Source: CAD feature listing. Evaluate the final solid. Frame: model axes, mm. Round coordinates to 2 decimals unless told otherwise and drop trailing zeros. Order: outer loops, then holes, each group sorted by start corner. A loop starts at its lowest first (then second) coordinate and runs counter-clockwise, first axis right, second up. Notation, with made-up numbers: (-29, 60.25) -> (19, 60.25) arc R14 ccw to (19, 75.25) -> close; hole circle Ø11 at (51.25, 50). An arc over 180 degrees is marked (long way). Write item = value, one per line. Start each with the question number.
(1) Cut plane B-B on x = -16. Return the cut outline in (y, z).
(2) Ray query, line 1 (Y direction, x = -49.5, z = 0.55); line 2 (Y direction, x = -12, z = 0.85); line 3 (Y direction, x = -76.5, z = 0.15). Return the intervals inside material, ascending.
(3) Contact query for flat-ended pins moving along their axis: pin 1 Ø1 at (y, z) = (76.5, 1) entering from +X; pin 2 Ø1 at (y, z) = (39, 1) entering from +X; pin 3 Ø1 at (y, z) = (20, 1.5) entering from -X. Output: stop coordinate, or through.
(4) Cut plane A-A on x = -49. Return the cut outline in (y, z).
(5) Cut plane C-C on y = 42. Give the number of separate pieces and of enclosed holes in the cut face, then the cut area to 3 significant figures.
from build123d import *

# Parameters (mm, degrees)
F2_DEPTH = 2
F3_W     = 2
F3_H     = 10
F3_H_2   = 7.419568
F4_DEPTH = 25
F6_DEPTH = 2
F7_W     = 5
F7_H     = 44.93185
F7_H_2   = 80.277377
F7_H_3   = 143.82022
F7_H_4   = 146.914949
F7_H_5   = 150.008155
F7_H_6   = 155.922672
F7_H_7   = 152.60311
F7_H_8   = 158.631397
F7_H_9   = 74.565352
F7_H_10  = 59.935174
F7_H_11  = 17.802537
F7_H_12  = 20.475702
F7_H_13  = 22.61665
F7_H_14  = 22.198746
F7_H_15  = 21.923671
F7_H_16  = 21.644043
F7_H_17  = 21.303791
F7_H_18  = 21.036336
F7_H_19  = 20.777645
F7_H_20  = 20.346487
F7_W_2   = 3
F7_H_21  = 20.140204
F8_DEPTH = 5


with BuildPart() as f2:
    # F1 (on Top) → F2 (new body)
    with BuildSketch(Plane.XY):
        with BuildLine():
            Line((-10.286918, 88.926369), (-80.9691, 88.926369))
            Line((-80.9691, 88.926369), (-80.9691, -91.073631))
            Line((-80.9691, -91.073631), (79.0309, -91.073631))
            Line((79.0309, -91.073631), (79.0309, -62.904311))
            Line((79.0309, -62.904311), (-0.788567, -58.895134))
            ThreePointArc((-0.788567, -58.895134), (-7.533175, -55.799151), (-10.286918, -48.907724))
            Line((-10.286918, -48.907724), (-10.286918, 88.926369))
        make_face()
    extrude(amount=F2_DEPTH)

    # F3 (on Top) → F4 (cut)
    with BuildSketch(Plane.XY):
        Polygon((-10.970959, -7.614357), (-20.367885, -11.034559), (-19.683845, -12.913944), (-10.286918, -9.493742), align=None)
        Polygon((-5.092329, -5.474711), (-10.970959, -7.614357), (-10.286918, -9.493742), (-4.408289, -7.354096), align=None)
        Polygon((-10.970959, 80.805754), (-20.367885, 77.385553), (-19.683845, 75.506168), (-10.286918, 78.926369), align=None)
        Polygon((-3.998845, 83.343396), (-10.970959, 80.805754), (-10.286918, 78.926369), (-3.314805, 81.464011), align=None)
        Polygon((-80.9691, 32.230381), (-71.572174, 28.810179), (-70.888133, 30.689565), (-80.28506, 34.109766), align=None)
        Polygon((-87.941213, 34.768023), (-80.9691, 32.230381), (-80.28506, 34.109766), (-87.257173, 36.647408), align=None)
        Polygon((-80.9691, -61.360746), (-71.572174, -64.780947), (-70.888133, -62.901562), (-80.28506, -59.48136), align=None)
        Polygon((-87.941213, -58.823104), (-80.9691, -61.360746), (-80.28506, -59.48136), (-87.257173, -56.943719), align=None)
        with Locations((75.0309, -67.753627)):
            Rectangle(F3_W, F3_H)
        with Locations((75.0309, -59.043843)):
            Rectangle(F3_W, F3_H_2)
    extrude(amount=F4_DEPTH, mode=Mode.SUBTRACT)

    # F5 (on Top) → F6 (join)
    with BuildSketch(Plane.XY):
        with BuildLine():
            Line((-84.190791, -61.073631), (-86.1691, -61.073631))
            ThreePointArc((-86.1691, -61.073631), (-87.583313, -61.659417), (-88.1691, -63.073631))
            Line((-88.1691, -63.073631), (-88.1691, -79.073631))
            ThreePointArc((-88.1691, -79.073631), (-87.583313, -80.487844), (-86.1691, -81.073631))
            Line((-86.1691, -81.073631), (-83.1691, -81.073631))
            Line((-83.1691, -81.073631), (-80.9691, -81.073631))
            Line((-80.9691, -81.073631), (-80.9691, -71.073631))
            Line((-80.9691, -71.073631), (-83.1691, -71.073631))
            Line((-83.1691, -71.073631), (-83.1691, -62.095322))
            ThreePointArc((-83.1691, -62.095322), (-83.468346, -61.372877), (-84.190791, -61.073631))
        make_face()
        with BuildLine():
            Line((-84.190791, 18.926369), (-86.1691, 18.926369))
            ThreePointArc((-86.1691, 18.926369), (-87.583313, 18.340583), (-88.1691, 16.926369))
            Line((-88.1691, 16.926369), (-88.1691, 0.926369))
            ThreePointArc((-88.1691, 0.926369), (-87.583313, -0.487844), (-86.1691, -1.073631))
            Line((-86.1691, -1.073631), (-83.1691, -1.073631))
            Line((-83.1691, -1.073631), (-80.9691, -1.073631))
            Line((-80.9691, -1.073631), (-80.9691, 8.926369))
            Line((-80.9691, 8.926369), (-83.1691, 8.926369))
            Line((-83.1691, 8.926369), (-83.1691, 17.904678))
            ThreePointArc((-83.1691, 17.904678), (-83.468346, 18.627123), (-84.190791, 18.926369))
        make_face()
        with BuildLine():
            Line((-84.190791, 83.926369), (-86.1691, 83.926369))
            ThreePointArc((-86.1691, 83.926369), (-87.583313, 83.340583), (-88.1691, 81.926369))
            Line((-88.1691, 81.926369), (-88.1691, 65.926369))
            ThreePointArc((-88.1691, 65.926369), (-87.583313, 64.512156), (-86.1691, 63.926369))
            Line((-86.1691, 63.926369), (-80.9691, 63.926369))
            Line((-80.9691, 63.926369), (-80.9691, 73.926369))
            Line((-80.9691, 73.926369), (-83.1691, 73.926369))
            Line((-83.1691, 73.926369), (-83.1691, 82.904678))
            ThreePointArc((-83.1691, 82.904678), (-83.468346, 83.627123), (-84.190791, 83.926369))
        make_face()
        with BuildLine():
            Line((-10.286918, 58.926369), (-9.800001, 58.926369))
            Line((-9.800001, 58.926369), (-8.086918, 58.926369))
            Line((-8.086918, 58.926369), (-7.600001, 58.926369))
            Line((-7.600001, 58.926369), (-5.086918, 58.926369))
            ThreePointArc((-5.086918, 58.926369), (-3.672705, 59.512156), (-3.086918, 60.926369))
            Line((-3.086918, 60.926369), (-3.086918, 76.926369))
            ThreePointArc((-3.086918, 76.926369), (-3.672705, 78.340583), (-5.086918, 78.926369))
            Line((-5.086918, 78.926369), (-7.065227, 78.926369))
            ThreePointArc((-7.065227, 78.926369), (-7.787672, 78.627123), (-8.086918, 77.904678))
            Line((-8.086918, 77.904678), (-8.086918, 68.926369))
            Line((-8.086918, 68.926369), (-10.286918, 68.926369))
            Line((-10.286918, 68.926369), (-10.286918, 58.926369))
        make_face()
        with BuildLine():
            Line((-10.286918, -21.073631), (-10.286918, -31.073631))
            Line((-10.286918, -31.073631), (-8.086918, -31.073631))
            Line((-8.086918, -31.073631), (-5.086918, -31.073631))
            ThreePointArc((-5.086918, -31.073631), (-3.672705, -30.487844), (-3.086918, -29.073631))
            Line((-3.086918, -29.073631), (-3.086918, -13.073631))
            ThreePointArc((-3.086918, -13.073631), (-3.672705, -11.659417), (-5.086918, -11.073631))
            Line((-5.086918, -11.073631), (-7.065227, -11.073631))
            ThreePointArc((-7.065227, -11.073631), (-7.787672, -11.372877), (-8.086918, -12.095322))
            Line((-8.086918, -12.095322), (-8.086918, -21.073631))
            Line((-8.086918, -21.073631), (-10.286918, -21.073631))
        make_face()
    extrude(amount=F6_DEPTH)

    # F7 (on Top) → F8 (cut)
    with BuildSketch(Plane.XY):
        with Locations((-73.4691, 61.460444)):
            Rectangle(F7_W, F7_H)
        with Locations((-72.413613, -17.006834)):
            Rectangle(F7_W, F7_H_2)
        with Locations((-65.4691, 12.016259)):
            Rectangle(F7_W, F7_H_3)
        with Locations((-57.4691, 10.468894)):
            Rectangle(F7_W, F7_H_4)
        with Locations((-49.4691, 8.922292)):
            Rectangle(F7_W, F7_H_5)
        with Locations((-33.4691, 5.965033)):
            Rectangle(F7_W, F7_H_6)
        with Locations((-41.4691, 7.624814)):
            Rectangle(F7_W, F7_H_7)
        with Locations((-25.4691, 4.61067)):
            Rectangle(F7_W, F7_H_8)
        with Locations((-16.4691, 34.384946)):
            Rectangle(F7_W, F7_H_9)
        with Locations((-16.4691, -47.720004)):
            Rectangle(F7_W, F7_H_10)
        with Locations((-8.4691, -71.7002)):
            Rectangle(F7_W, F7_H_11)
        with Locations((-0.4691, -73.37924)):
            Rectangle(F7_W, F7_H_12)
        with Locations((7.5309, -74.765306)):
            Rectangle(F7_W, F7_H_13)
        with Locations((15.5309, -74.974258)):
            Rectangle(F7_W, F7_H_14)
        with Locations((23.5309, -75.111795)):
            Rectangle(F7_W, F7_H_15)
        with Locations((31.5309, -75.25161)):
            Rectangle(F7_W, F7_H_16)
        with Locations((39.5309, -75.421735)):
            Rectangle(F7_W, F7_H_17)
        with Locations((47.5309, -75.555463)):
            Rectangle(F7_W, F7_H_18)
        with Locations((55.5309, -75.684809)):
            Rectangle(F7_W, F7_H_19)
        with Locations((63.5309, -75.900387)):
            Rectangle(F7_W, F7_H_20)
        with Locations((70.5309, -76.003529)):
            Rectangle(F7_W_2, F7_H_21)
    extrude(amount=F8_DEPTH, mode=Mode.SUBTRACT)


solid = f2.part
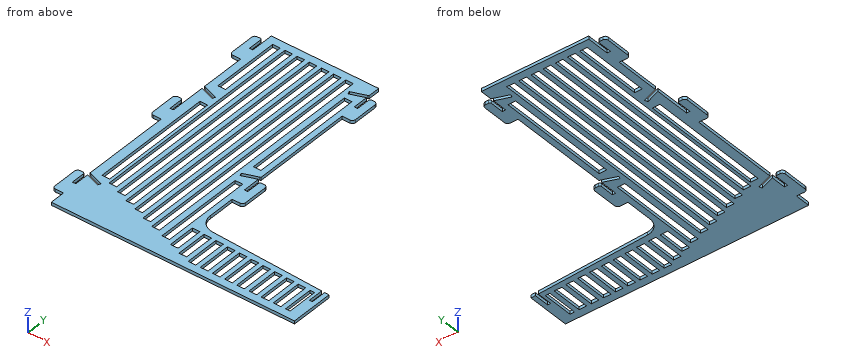
Evaluation:
q1.outline = (-91.07, 0) -> (-77.69, 0) -> (-77.69, 2) -> (-91.07, 2) -> close; (-17.75, 0) -> (-11.57, 0) -> (-11.57, 2) -> (-17.75, 2) -> close; (-9.44, 0) -> (-2.9, 0) -> (-2.9, 2) -> (-9.44, 2) -> close; (71.67, 0) -> (76.85, 0) -> (76.85, 2) -> (71.67, 2) -> close; (78.98, 0) -> (88.93, 0) -> (88.93, 2) -> (78.98, 2) -> close
q2.line_1 = -91.07 to -66.08, 83.93 to 88.93
q2.line_2 = -91.07 to -10.12, -7.99 to 78.3, 80.43 to 88.93
q2.line_3 = -91.07 to -62.99, -60.86 to 30.6, 32.73 to 88.93
q3.pin_1 = -3.09
q3.pin_2 = -10.29
q3.pin_3 = -80.97
q4.outline = (-91.07, 0) -> (-66.08, 0) -> (-66.08, 2) -> (-91.07, 2) -> close; (83.93, 0) -> (88.93, 0) -> (88.93, 2) -> (83.93, 2) -> close
q5.separate_pieces = 9
q5.enclosed_holes = 0
q5.area = 61.4 mm^2
